Verification items for the finished model (mm, model axes). Coordinates: 2 decimals unless noted, no trailing zeros. Order: outer loops, then holes, each group sorted by start corner. A loop starts at its lowest first (then second) coordinate and runs counter-clockwise, first axis right, second up. Notation, with made-up numbers: (7, 45.5) - (15, 45.5) arc R17 cw to (15, 52.5) - close; hole circle Ø6 at (62, 70.5). An arc over 180 degrees is marked (long way). Answer as CSV lines item,"result". Start each with the question number.
1. Section check A-A (x = 0). Record the cut outline in (y, z), and give its area (3 significant figures).
2. Section check C-C (z = 0.85). Record the cut outline in (x, y).
3. Material ranges on L1, parallel to Y at x = 0, z = 2.3; L2, parallel to X at y = 1, z = 0.4; L3, parallel to Y at x = -14, z = 1.8, recorded low to high. Write a range as [from, to].
4. Go/stop test with flat-tipped pins: pin 1 (3 mm diameter, centred on x = 0, y = 0, fed in from -Z); pin 2 (1.5 mm diameter, centred on y = 22.5, z = 1, fed in from -X); pin 3 (1.5 mm diameter, centred on x = -0.5, z = 0.5, fed in from -Y); pin 4 (1.5 mm diameter, centred on x = -49, z = 2.5, fed in from +Y). Record where each tip stops, or that it passes through.
5. Mould release check, pull along Y, two halves, no side actions. Record for faces 1 (the flat face through (-30.81, 50.5, 1.48)), 2 (the flat face through (-30, 38, 3)), 3 (the cylindrical face through (-15.88, 21.18, 1.48)): pulls with the +Y half, pulls with the -Y half, needs draft (parallel to the pull), parting line crosses it, or undercut.
6. Section check D-D (y = 34). Record the cut outline in (x, z), and give its area (3 significant figures).
from build123d import *

# Parameters (mm, degrees)
SKETCH1_R           = 2.5
SKETCH1_R_2         = 1.500000002
BOSS_EXTRUDE1_DEPTH = 3


with BuildPart() as part:
    # Sketch1 → Boss-Extrude1 (new body)
    with BuildSketch(Plane.XY):
        with BuildLine():
            Line((-65.41272675, 89.25730784), (-69.445670133, 86.301742297))
            Line((-69.445670133, 86.301742297), (-9.152133067, 4.0296973))
            ThreePointArc((-9.152133067, 4.0296973), (5.911131085, -8.065886764), (-1.086246302, 9.940828385))
            Line((-1.086246302, 9.940828385), (-61.379783368, 92.212873382))
            Line((-61.379783368, 92.212873382), (-65.41272675, 89.25730784))
        make_face()
        Circle(SKETCH1_R, mode=Mode.SUBTRACT)
        with Locations((-14.777827712, 20.164716911)):
            Circle(SKETCH1_R_2, mode=Mode.SUBTRACT)
    extrude(amount=BOSS_EXTRUDE1_DEPTH)


solid = part.part
Evaluation:
1,outline,"(-10, 0) - (-2.5, 0) - (-2.5, 3) - (-10, 3) - close; (2.5, 0) - (10, 0) - (10, 3) - (2.5, 3) - close"
1,area,"45.0 mm²"
2,outline,"(-69.45, 86.3) - (-9.15, 4.03) arc R10 ccw (long way) to (-1.09, 9.94) - (-61.38, 92.21) - close; hole circle Ø3 at (-14.78, 20.16); hole circle Ø5 at (0, 0)"
3,L1,"y = [-10, -2.5], [2.5, 10]"
3,L2,"x = [-9.95, -2.29], [2.29, 9.95]"
3,L3,"y = [10.64, 18.88], [21.45, 27.56]"
4,pin 1,"passes through"
4,pin 2,"stops at x = -23.24"
4,pin 3,"stops at y = -10"
4,pin 4,"stops at y = 76.34"
5,face 1,"pulls with the +Y half"
5,face 2,"needs draft"
5,face 3,"undercut"
6,outline,"(-31.12, 0) - (-18.72, 0) - (-18.72, 3) - (-31.12, 3) - close"
6,area,"37.2 mm²"
